Work out the finished part from the listing and answer in its coordinate system (mm). Round coordinates to 2 decimals unless told otherwise and drop trailing zeros. Loops run counter-clockwise (first coordinate to the right, second up) from the corner with the lowest first, then second, coordinate; pieces in that order, holes last. Notation, with made-up numbers: (52.25, 1) - (79.25, 1) arc R24 cw to (79.25, 20) - close; hole circle Ø3 at (-39, 70). An arc over 180 degrees is marked (long way). Answer as CSV lines item,"result". Start each with the question number.
Q1. Section C-C on x = -13.25 is taken. Write down the section's boundary in (y, z), then the cut area to 4 significant figures.
Q2. Section D-D on y = -3.5 is taken. Write down the section's boundary in (x, z), then the cut area to 3 significant figures.
Q3. Section B-B on x = -81.5 is taken. Write down the section's boundary in (y, z).
Q4. Straight lines are drawn through the part: L1, parallel to X at y = -3.95, z = 13.5; L2, parallel to Z at x = -13.25, y = -1.5; L3, parallel to Z at x = -81.5, y = -1.9. For each, find the intervals that lie inside material, in ascending order. Write a range as [from, to].
Q5. The mould has two halves that part along Z. Classify faces 1 (the face through (-89.953, -2.465, 13.395)), 2 (the face through (-54, 0, 54)), 3 (the face through (-54, -2, 0)): +Z half, -Z half, draft (parallel to the pull), parting line (faces both ways), or undercut.
Q6. Section A-A on z = 13.25 is taken. Write down the section's boundary in (x, y).
```python
from build123d import *

# Parameters (mm, degrees)
F0_W     = 106.5
F0_H     = 106.5
F1_DEPTH = 5
F3_D     = 6.6
F5_D     = 16


with BuildPart() as f1:
    # F0 (on Front) → F1 (new body)
    with BuildSketch(Plane.XZ):
        with Locations((-53.25, 53.25)):
            Rectangle(F0_W, F0_H)
    extrude(amount=F1_DEPTH)

    # F3 (through all)
    with Locations(Plane.XZ.offset(5)):
        with Locations((-93.25, 93.25), (-93.25, 13.25), (-13.25, 13.25), (-13.25, 93.25)):
            Hole(F3_D / 2)

    # F5 (through all)
    with Locations(Plane.XZ.offset(5)):
        with Locations((-81.5, 53.25)):
            Hole(F5_D / 2)


solid = f1.part
```
Findings:
1,outline,"(-5, 0) - (0, 0) - (0, 9.95) - (-5, 9.95) - close; (-5, 16.55) - (0, 16.55) - (0, 89.95) - (-5, 89.95) - close; (-5, 96.55) - (0, 96.55) - (0, 106.5) - (-5, 106.5) - close"
1,area,"466.5 mm^2"
2,outline,"(-106.5, 0) - (0, 0) - (0, 106.5) - (-106.5, 106.5) - close; hole circle Ø6.6 at (-93.25, 13.25); hole circle Ø6.6 at (-93.25, 93.25); hole circle Ø16 at (-81.5, 53.25); hole circle Ø6.6 at (-13.25, 13.25); hole circle Ø6.6 at (-13.25, 93.25)"
2,area,"11,000 mm^2"
3,outline,"(-5, 0) - (0, 0) - (0, 45.25) - (-5, 45.25) - close; (-5, 61.25) - (0, 61.25) - (0, 106.5) - (-5, 106.5) - close"
4,L1,"x = [-106.5, -96.54], [-89.96, -16.54], [-9.96, 0]"
4,L2,"z = [0, 9.95], [16.55, 89.95], [96.55, 106.5]"
4,L3,"z = [0, 45.25], [61.25, 106.5]"
5,face 1,"undercut"
5,face 2,"draft"
5,face 3,"-Z half"
6,outline,"(-106.5, -5) - (-96.55, -5) - (-96.55, 0) - (-106.5, 0) - close; (-89.95, -5) - (-16.55, -5) - (-16.55, 0) - (-89.95, 0) - close; (-9.95, -5) - (0, -5) - (0, 0) - (-9.95, 0) - close"
